Geometry check sheet. Reference: the model listing, model coordinates, mm. Face numbers are marked on the shaded views. A direction names the side the tool comes from. Coordinates: 2 decimals unless noted, no trailing zeros. Loops run counter-clockwise (first coordinate to the right, second up) from the corner with the lowest first, then second, coordinate; pieces in that order, holes last. Notation, with made-up numbers: (52, -36.5) - (104, -36.5) arc R22 cw to (104, -17.5) - close; hole circle Ø9 at (-39, -5). An arc over 180 degrees is marked (long way). One line per item, written item: value.
from build123d import *

# Parameters (mm, degrees)
SKETCH1_W           = 150
SKETCH1_H           = 20
BOSS_EXTRUDE1_DEPTH = 10
BOSS_EXTRUDE2_DEPTH = 10
BOSS_EXTRUDE3_DEPTH = 23
SKETCH6_R           = 3
CUT_EXTRUDE2_DEPTH  = 46


with BuildPart() as part:
    # Sketch1 → Boss-Extrude1 (new, symmetric)
    with BuildSketch(Plane(origin=(0, 0, 0), x_dir=(1, 0, 0), z_dir=(0, 1, 0))):
        Rectangle(SKETCH1_W, SKETCH1_H)
    extrude(amount=BOSS_EXTRUDE1_DEPTH, both=True)

    # Sketch2 → Boss-Extrude2 (add, symmetric)
    with BuildSketch(Plane.XY):
        Polygon((-75, 10), (75, 10), (75, 28.417684135), align=None)
    extrude(amount=BOSS_EXTRUDE2_DEPTH, both=True)

    # Sketch3 → Boss-Extrude3 (add, symmetric)
    with BuildSketch(Plane.XY):
        Polygon((75, 28.417684135), (-75, 10), (-73.772154391, 0), (76.227845609, 18.417684135), align=None)
    extrude(amount=BOSS_EXTRUDE3_DEPTH, both=True)

    # Sketch6 → Cut-Extrude2 (cut)
    with BuildSketch(Plane(origin=(-2.323519743, 18.923549716, 0), x_dir=(0.9925461516413229, 0.12186934340514101, 0), z_dir=(-0.12186934340514102, 0.992546151641323, 0))):
        with Locations(Location((-54.222267939, 16.5, 0), (0, 0, 180))):
            Circle(SKETCH6_R)
        with Locations(Location((58.90420588, 16.5, 0), (0, 0, 180))):
            Circle(SKETCH6_R)
        with Locations(Location((58.90420588, -16.5, 0), (0, 0, 180))):
            Circle(SKETCH6_R)
        with Locations(Location((-54.222267939, -16.5, 0), (0, 0, 180))):
            Circle(SKETCH6_R)
    extrude(amount=-CUT_EXTRUDE2_DEPTH, mode=Mode.SUBTRACT)


solid = part.part
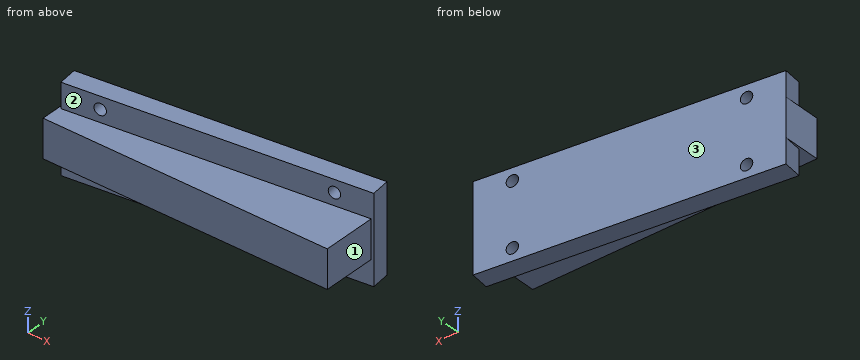
(1) Cross-section at A-A on z = -18. Record the cut outline in (x, y), and give its area (3 significant figures).
Reply:
outline: (-75, 10) - (-73.77, 0) - (-57.49, 2) - (-58.72, 12) - close; (-53.56, 12.63) - (-52.34, 2.63) - (54.79, 15.79) - (53.56, 25.79) - close; (58.72, 26.42) - (59.95, 16.42) - (76.23, 18.42) - (75, 28.42) - close
area: 1,420 mm2
(2) Cross-section at C-C on z = 7. Record the cut outline in (x, y), and give its area (3 significant figures).
Reply:
outline: (-75, -10) - (75, -10) - (75, 18.27) - (76.23, 18.42) - (75, 28.42) - (-75, 10) - close
area: 4,390 mm2
(3) Access from +Z, -Z, +X, -X, +Y, -Y to the whole of each face (thin tool, end or side, straight path). Record for the marked faces 1, 2 and 3.
Reply:
face 1: +Z, -Z, +X, -Y
face 2: +X, -Y
face 3: +Z, -Z, -X, +Y
(4) Material ranges on probe 1 along Z at (x, y) = (25, 4); probe 2 along X at (y, z) = (7, 7); probe 3 along Y at (x, z) = (-28.5, 9), recorded low to high. Write a range as from..to.
Reply:
probe 1: -10..10
probe 2: -75..75
probe 3: -10..15.71
(5) Cross-section at D-D on y = -2. Record the cut outline in (x, z), and give its area (3 significant figures).
Reply:
outline: (-75, -10) - (75, -10) - (75, 10) - (-75, 10) - close
area: 3,000 mm2
(6) Go/stop test with flat-tipped pins: pin 1 Ø2 at (y, z) = (20.5, -10.5) entering from +X; pin 2 Ø22 at (y, z) = (-0.5, -0.5) entering from +X; pin 3 Ø8 at (x, z) = (22, 1.5) entering from +Y. Record where each tip stops, or that it passes through.
Reply:
pin 1: x = 76.09
pin 2: x = 75
pin 3: y = 22.4
(7) Cross-section at B-B on x = -30.5. Record the cut outline in (y, z).
Reply:
outline: (-10, -10) - (5.31, -10) - (5.31, -23) - (15.46, -23) - (15.46, 23) - (5.31, 23) - (5.31, 10) - (-10, 10) - close
